Design review of the part shown in the three views and the two pictorial views. Dimensions are in mm from the part's minimum x, y and z. A direction names the side the tool comes from. Round coordinates to 2 decimals unless told otherwise and drop trailing zeros. Loops run counter-clockwise (first coordinate to the right, second up) from the corner with the lowest first, then second, coordinate; pieces in that order, holes last. Notation, with made-up numbers: (29.25, -26.5) -> (44.25, -26.5) arc R32 ccw to (44.25, 3.5) -> close; hole circle Ø10 at (-7, 7.5). An arc over 180 degrees is marked (long way). Use a Markdown table: item, result. Add a question column.
1) Consider section A-A on y = 30. Give the boundary of the cut face in (x, z) (1 decimal).
2) Consider section D-D on x = 148.5. Give the boundary of the cut face in (y, z), plus the area to 3 significant figures.
3) For the marked faces 1, 2 and 3, list the 3-axis set-ups (+Z, -Z, +X, -X, +Y, -Y) from which the entire face can be reached by the end or side of a thin tool; tool diameter is ignored.
4) Consider section B-B on x = 73. Give the boundary of the cut face in (y, z).
5) Consider section C-C on z = 12. Give the boundary of the cut face in (x, y) (1 decimal).
6) Insertion check: pin 1 (4 mm diameter, centred on x = 44.5, z = 3.5, fed in from -Y); pin 2 (1 mm diameter, centred on y = 19, z = 16.5, fed in from +X); pin 3 (5 mm diameter, centred on x = 149.5, z = 9, fed in from +Y) (1 decimal); pin 4 (5 mm diameter, centred on x = 154.5, y = 50.5, fed in from +Z). Each pin has a flat end and moves straight along its axis. Give the tip position at first contact, or say it passes through.
7) Mouldability with a two-part tool opening along Y and no side actions: class the marked faces 4, 5 and 6 as released by +Y, released by -Y, zero draft, split by the parting line, or undercut.
8) Wall thickness on probe 1 along X at (y, z) = (29, 12.25) (1 decimal); probe 2 along X at (y, z) = (34, 15.75) (1 decimal); probe 3 along Y at (x, z) = (88.5, 5.5): over which ranges is each line inside the solid? List them lowest first.
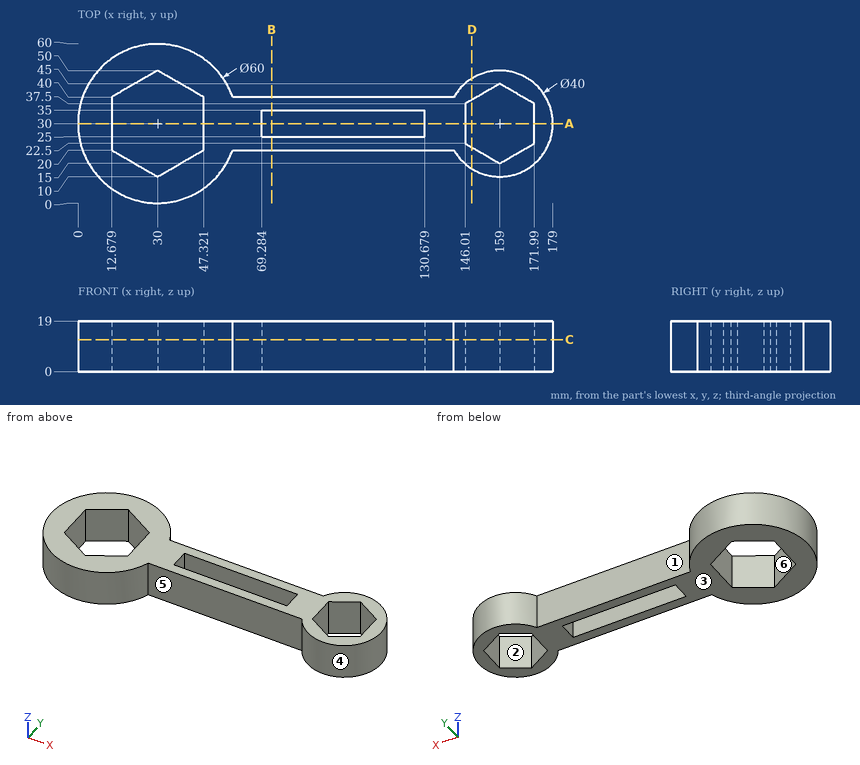
Result set:
| question | item | result |
|---|---|---|
| 1 | outline | (0, 0) -> (12.7, 0) -> (12.7, 19) -> (0, 19) -> close; (47.3, 0) -> (69.3, 0) -> (69.3, 19) -> (47.3, 19) -> close; (130.7, 0) -> (146, 0) -> (146, 19) -> (130.7, 19) -> close; (172, 0) -> (179, 0) -> (179, 19) -> (172, 19) -> close |
| 2 | outline | (12.98, 0) -> (21.06, 0) -> (21.06, 19) -> (12.98, 19) -> close; (38.94, 0) -> (47.02, 0) -> (47.02, 19) -> (38.94, 19) -> close |
| 2 | area | 307 mm2 |
| 3 | face 1 | +Z, -Z, +Y |
| 3 | face 2 | +Z, -Z |
| 3 | face 3 | -Z, +X, -X, +Y, -Y |
| 4 | outline | (20, 0) -> (25, 0) -> (25, 19) -> (20, 19) -> close; (35, 0) -> (40, 0) -> (40, 19) -> (35, 19) -> close |
| 5 | outline | (58.3, 20) -> (141.7, 20) arc R20 ccw (long way) to (141.7, 40) -> (58.3, 40) arc R30 ccw (long way) to start; hole (12.7, 20) -> (30, 10) -> (47.3, 20) -> (47.3, 40) -> (30, 50) -> (12.7, 40) -> close; hole (69.3, 25) -> (130.7, 25) -> (130.7, 35) -> (69.3, 35) -> close; hole (146, 22.5) -> (159, 15) -> (172, 22.5) -> (172, 37.5) -> (159, 45) -> (146, 37.5) -> close |
| 6 | pin 1 | y = 2.73 |
| 6 | pin 2 | x = 176.02 |
| 6 | pin 3 | y = 48.7 |
| 6 | pin 4 | z = 19 |
| 7 | face 4 | split by the parting line |
| 7 | face 5 | released by -Y |
| 7 | face 6 | undercut |
| 8 | probe 1 | 0 to 12.7, 47.3 to 69.3, 130.7 to 146, 172 to 179 |
| 8 | probe 2 | 0.3 to 12.7, 47.3 to 69.3, 130.7 to 146, 172 to 178.6 |
| 8 | probe 3 | 20 to 25, 35 to 40 |
